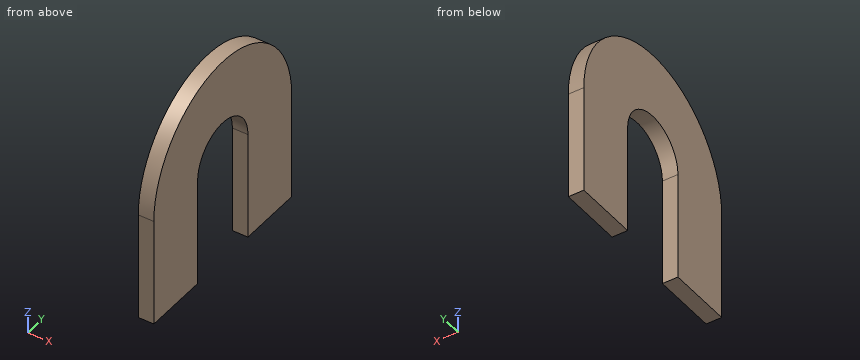
```python
from build123d import *

# Parameters (mm, degrees)
PAD010_DEPTH = 12


with BuildPart() as support_hook:
    # Sketch023 → Pad010 (new body)
    with BuildSketch(Plane.YZ):
        with BuildLine():
            Line((-28.75, 0), (-78.75, 0))
            Line((-78.75, 0), (-78.75, 84))
            ThreePointArc((78.75, 84), (0, 162.75), (-78.75, 84))
            Line((78.75, 0), (78.75, 84))
            Line((28.75, 0), (78.75, 0))
            Line((28.75, 84), (28.75, 0))
            ThreePointArc((28.75, 84), (0, 112.75), (-28.75, 84))
            Line((-28.75, 0), (-28.75, 84))
        make_face()
    extrude(amount=PAD010_DEPTH)


with BuildPart() as support_hook_1:
    # Body011 placement: moved
    add(support_hook.part.moved(Location((200, 200, 0))))


with BuildPart() as part_mirroring007:
    # Part__Mirroring007: instance of support_hook
    add(support_hook_1.part.mirror(Plane(origin=(0, 0, 0), x_dir=(1, 0, 0), z_dir=(0, 1, 0))))


with BuildPart() as part_mirroring008:
    # Part__Mirroring008: instance of Part__Mirroring007
    add(part_mirroring007.part.mirror(Plane(origin=(0, 0, 0), x_dir=(0, -1, 0), z_dir=(1, 0, 0))))


solid = part_mirroring008.part
```
Could you check a few things on this model? Use its own coordinates, in mm. Give positions to 0.01 mm unless a question says otherwise; leave off trailing zeros. Loops run counter-clockwise (first coordinate to the right, second up) from the corner with the lowest first, then second, coordinate; pieces in that order, holes last. Notation, with made-up numbers: (44.25, -24.75) - (76.25, -24.75) arc R13 ccw to (76.25, -10.75) - close; hole circle Ø8 at (48, 1). An arc over 180 degrees is marked (long way). Answer in a Markdown table with one row per item. Add a question column.
Q1. If we section it at D-D (y = -200): List the corners of the cut face in (x, z) for me, plus the area to 3 significant figures.
Q2. For pin 1 (5 mm diameter, centred on x = -202, z = 94.5, fed in from -Y); pin 2 (5 mm diameter, centred on x = -208, z = 140.5, fed in from +Y); pin 3 (1 mm diameter, centred on x = -202, z = 105, fed in from -Y); pin 4 (1.5 mm diameter, centred on x = -203.5, y = -240, fed in from -Z), each with a flat end and sliding along its axis, tell me the tip position at first contact or that it passes through.
Q3. If we section it at A-A (z = 14): List the corners of the cut face in (x, y) for me.
Q4. If we section it at C-C (z = 109): List the corners of the cut face in (x, y) for me, plus the area to 3 significant figures.
Q5. Please list where these lines run through material, in increasing order: L1, parallel to Y at x = -208.5, z = 7; L2, parallel to Y at x = -209, z = 149; L3, parallel to Y at x = -202.25, z = 105.5. Write a range as from..to.
Q6. If we section it at B-B (x = -208.5): List the corners of the cut face in (y, z) for me.
The answers:
| question | item | result |
|---|---|---|
| 1 | outline | (-212, 112.75) - (-200, 112.75) - (-200, 162.75) - (-212, 162.75) - close |
| 1 | area | 600 mm^2 |
| 2 | pin 1 | stops at y = -278.34 |
| 2 | pin 2 | stops at y = -142.68 |
| 2 | pin 3 | stops at y = -276.03 |
| 2 | pin 4 | stops at z = 0 |
| 3 | outline | (-212, -278.75) - (-200, -278.75) - (-200, -228.75) - (-212, -228.75) - close; (-212, -171.25) - (-200, -171.25) - (-200, -121.25) - (-212, -121.25) - close |
| 4 | outline | (-212, -274.68) - (-200, -274.68) - (-200, -214.2) - (-212, -214.2) - close; (-212, -185.8) - (-200, -185.8) - (-200, -125.32) - (-212, -125.32) - close |
| 4 | area | 1,450 mm^2 |
| 5 | L1 | y = -278.75..-228.75, -171.25..-121.25 |
| 5 | L2 | y = -244.46..-155.54 |
| 5 | L3 | y = -275.76..-219.09, -180.91..-124.24 |
| 6 | outline | (-278.75, 0) - (-228.75, 0) - (-228.75, 84) arc R28.75 cw to (-171.25, 84) - (-171.25, 0) - (-121.25, 0) - (-121.25, 84) arc R78.75 ccw to (-278.75, 84) - close |
